Here's how the part is built. I have some questions about the finished solid (model axes, mm). A direction names the side the tool comes from. Coordinates: 2 decimals unless noted, no trailing zeros. Write each loop counter-clockwise with the first axis right and the second up, starting at its lowest first coordinate (ties: lowest second). Pieces come first, ordered by that corner, then holes. Notation, with made-up numbers: (38, 73) -> (65, 73) arc R11 ccw to (65, 88) -> close; hole circle Ø6 at (-8, 32). An arc over 180 degrees is marked (long way). Put each result on its own line as item: value.
```python
from build123d import *

# Parameters (mm, degrees)
SMUSSO1_SIZE              = 0.5
SCHIZZO2_R                = 1.5
TAGLIO_ESTRUSIONE1_DEPTH  = 10
FORO_PER_VITE_M2_2_REACH  = 18.726
FORO_PER_VITE_M2_2_BORE_R = 1.2


with BuildPart() as part:
    # Schizzo1 → Rivoluzione1 (revolve)
    with BuildSketch(Plane.XY, mode=Mode.PRIVATE) as rivoluzione1_sk:
        Polygon((-7, 14), (-7, 6.5), (-4.25, 6.5), (-4.25, 0), (0, 0), (0, 14), align=None)
    revolve(rivoluzione1_sk.sketch.rotate(Axis((0, 0, 0), (0, 1, 0)), 270), axis=Axis((0, 0, 0), (0, 1, 0)))

    # Smusso1
    smusso1_edges = [part.edges().sort_by_distance(p)[0] for p in [
        (0, 14, 7),
    ]]
    chamfer(smusso1_edges, length=SMUSSO1_SIZE)

    # Schizzo2 → Taglio-Estrusione1 (cut)
    with BuildSketch(Plane(origin=(0, 0, 0), x_dir=(-1, 0, 0), z_dir=(0, -1, 0))):
        with Locations(Location((0, 0, 0), (0, 0, 90))):
            Circle(SCHIZZO2_R)
    extrude(amount=-TAGLIO_ESTRUSIONE1_DEPTH, mode=Mode.SUBTRACT)

    # Foro per Vite M2-2 bore (on position points) → Foro per Vite M2-2 (cut, up to next)
    with BuildSketch(Plane(origin=(0.020038274, 3.80568373, 4.249952761), x_dir=(0.999988884854, 0, -0.004714888012), z_dir=(0.004714888012, 0, 0.999988884854)), mode=Mode.PRIVATE) as foro_per_vite_m2_2_sk1:
        Circle(FORO_PER_VITE_M2_2_BORE_R)
    foro_per_vite_m2_2_tool1 = extrude(foro_per_vite_m2_2_sk1.sketch, amount=-FORO_PER_VITE_M2_2_REACH, mode=Mode.PRIVATE) & part.part
    add(foro_per_vite_m2_2_tool1.solids().sort_by_distance((0.020038, 3.805684, 4.249953))[0], mode=Mode.SUBTRACT)


solid = part.part
```
Item 1: Please list where these lines run through material, in increasing order: line 1 along X through (y, z) = (7.25, 0); line 2 along X through (y, z) = (3, 0); line 3 along Y through (x, z) = (-2.75, 4.5). Write a range as from..to.
Output:
line 1: x = -7..-1.5, 1.5..7
line 2: x = -4.25..-1.5, 1.5..4.25
line 3: y = 6.5..14
Item 2: Which directions (+Z, -Z, +X, -X, +Y, -Y) give clear straight access to the entire face, cutting with the end or side of a thin tool? Please do faces 1 (the flat face through (5, 6.5, 0)), 2 (the flat face through (0, 0, -2)).
Output:
face 1: -Y
face 2: +Z, -Z, +X, -X, -Y
Item 3: Imagine slicing it at A-A on z = 0. Write out the boundary of the cut face in (x, y).
Output:
outline: (-7, 6.5) -> (-4.25, 6.5) -> (-4.25, 0) -> (-1.5, 0) -> (-1.5, 10) -> (1.5, 10) -> (1.5, 0) -> (4.25, 0) -> (4.25, 6.5) -> (7, 6.5) -> (7, 13.5) -> (6.5, 14) -> (-6.5, 14) -> (-7, 13.5) -> close
Item 4: For P1, Ø8, axis at y = 11.5, z = -4.5, coming from the +X side; P2, Ø4, axis at y = 1.5, z = -1, coming from the -X side; P3, Ø2.5, axis at x = 0, z = 0, coming from the -Y side, each with a flat end and sliding along its axis, tell me the tip position at first contact or that it passes through.
Output:
P1: stops at x = 6.98
P2: stops at x = -4.25
P3: stops at y = 10
Item 5: If we mould it in two halves opening along Z, with no side actions, what happens to faces 3 (the cylindrical face through (6.834, 9.951, 1.517)), 4 (the flat face through (0, 10, 0))? For each: released by +Z, released by -Z, zero draft, split by the parting line, or undercut.
Output:
face 3: split by the parting line
face 4: undercut
Item 6: Imagine slicing it at B-B on y = 2. Write out the boundary of the cut face in (x, z), then the cut area to 3 significant figures.
Output:
outline: circle Ø8.5 at (0, 0); hole circle Ø3 at (0, 0)
area: 49.7 mm²
